Here's how the part is built. I have some questions about the finished solid (model axes, mm). A direction names the side the tool comes from. Round coordinates to 2 decimals unless told otherwise and drop trailing zeros. Order: outer loops, then holes, each group sorted by start corner. A loop starts at its lowest first (then second) coordinate and runs counter-clockwise, first axis right, second up. Notation, with made-up numbers: M -36.75,4.5 L 6.25,4.5 A19 cw 6.25,28.5 Z; hole C -28,48.5 d9. An arc over 180 degrees is marked long. Write each question's results on one line, items separated by ' | '. Start each with the question number.
```python
from build123d import *

# Parameters (mm, degrees)
EXTRUDE_1_DEPTH          = 2
SKETCH_1_3_W             = 2.1
SKETCH_1_3_H             = 8.1
CUT_EXTRUDE_1_DEPTH      = 31.615900009
SKETCH_2_R               = 1.55
SKETCH_2_R_2             = 6
CUT_EXTRUDE_2_DEPTH      = 10
FILLET_1_R               = 10
SKETCH_4_R               = 0.4
CUT_EXTRUDE_3_DEPTH      = 10
PATTERN_CIRCULAR_1_COUNT = 5
PATTERN_CIRCULAR_1_ANGLE = 240
FILLET_2_R               = 0.3


with BuildPart() as part:
    # 草图1 → 凸台-拉伸1 (new body)
    with BuildSketch(Plane(origin=(0, 0, 0), x_dir=(1, 0, 0), z_dir=(0, 1, 0))):
        Polygon((20, -11.547005384), (20, 11.547005384), (0, 23.094010768), (-20, 11.547005384), (-20, -11.547005384), (0, -23.094010768), align=None)
    extrude(amount=EXTRUDE_1_DEPTH)

    # 草图1<3> → 切除-拉伸1 (cut, through all)
    with BuildSketch(Plane(origin=(0, 0, 0), x_dir=(1, 0, 0), z_dir=(0, 1, 0))):
        Polygon((8.091952768, -5.884326674), (15.106758538, -9.934326674), (16.156758538, -8.115673326), (9.141952768, -4.065673326), align=None)
        with Locations((0, -14)):
            Rectangle(SKETCH_1_3_W, SKETCH_1_3_H)
        Polygon((-8.091952768, -5.884326674), (-15.106758538, -9.934326674), (-16.156758538, -8.115673326), (-9.141952768, -4.065673326), align=None)
        Polygon((-9.141952768, 4.065673326), (-16.156758538, 8.115673326), (-15.106758538, 9.934326674), (-8.091952768, 5.884326674), align=None)
        Polygon((8.091952768, 5.884326674), (15.106758538, 9.934326674), (16.156758538, 8.115673326), (9.141952768, 4.065673326), align=None)
    extrude(amount=CUT_EXTRUDE_1_DEPTH, mode=Mode.SUBTRACT)

    # 草图2 → 切除-拉伸2 (cut)
    with BuildSketch(Plane(origin=(0, 2, 0), x_dir=(1, 0, 0), z_dir=(0, 1, 0))):
        with Locations(Location((15, 0, 0), (0, 0, 270))):
            Circle(SKETCH_2_R)
        with Locations(Location((0, 0, 0), (0, 0, 270))):
            Circle(SKETCH_2_R_2)
        with Locations(Location((7.5, -12.990381057, 0), (0, 0, 270))):
            Circle(SKETCH_2_R)
        with Locations(Location((-7.5, -12.990381057, 0), (0, 0, 270))):
            Circle(SKETCH_2_R)
        with Locations(Location((-15, 0, 0), (0, 0, 270))):
            Circle(SKETCH_2_R)
        with Locations(Location((-7.5, 12.990381057, 0), (0, 0, 270))):
            Circle(SKETCH_2_R)
        with Locations(Location((7.5, 12.990381057, 0), (0, 0, 270))):
            Circle(SKETCH_2_R)
    extrude(amount=-CUT_EXTRUDE_2_DEPTH, mode=Mode.SUBTRACT)

    # 圆角1
    fillet_1_edges = [part.edges().sort_by_distance(p)[0] for p in [
        (20, 1, -11.547005384),
        (20, 1, 11.547005384),
        (0, 1, 23.094010768),
        (-20, 1, 11.547005384),
        (-20, 1, -11.547005384),
        (0, 1, -23.094010768),
    ]]
    fillet(fillet_1_edges, radius=FILLET_1_R)

    # 草图4 → 切除-拉伸3 (cut)
    with BuildSketch(Plane(origin=(0, 2, 0), x_dir=(1, 0, 0), z_dir=(0, 1, 0))):
        with Locations((15.00323092, 9.547956343)):
            Circle(SKETCH_4_R)
        with Locations((15.770388208, 8.219200944)):
            Circle(SKETCH_4_R)
        with Locations((8.478323098, 5.780799056)):
            Circle(SKETCH_4_R)
        with Locations((9.245480386, 4.452043657)):
            Circle(SKETCH_4_R)
    cut_extrude_3 = extrude(amount=-CUT_EXTRUDE_3_DEPTH, mode=Mode.SUBTRACT)

    # 阵列(圆周)1: 切除-拉伸3 ×5 about axis
    pattern_circular_1_axis = Axis((0, 0, 0), (0, -1, 0))
    for i in range(1, PATTERN_CIRCULAR_1_COUNT):
        add(cut_extrude_3.rotate(pattern_circular_1_axis, i * PATTERN_CIRCULAR_1_ANGLE / (PATTERN_CIRCULAR_1_COUNT - 1)), mode=Mode.SUBTRACT)

    # 圆角2
    fillet_2_edges = [part.edges().sort_by_distance(p)[0] for p in [
        (8.37479548, 1, -5.394428725),
        (8.859110055, 1, -4.555571275),
        (14.61686059, 1, -9.651483961),
        (15.873915826, 1, -8.605571275),
        (15.389601251, 1, -9.444428725),
        (15.66686059, 1, -7.832830614),
        (9.631850716, 1, -4.348516039),
        (8.581850716, 1, -6.167169386),
        (-8.859110055, 1, -4.555571275),
        (-8.37479548, 1, -5.394428725),
        (-15.66686059, 1, -7.832830614),
        (-15.389601251, 1, -9.444428725),
        (-8.859110055, 1, 4.555571275),
        (-8.37479548, 1, 5.394428725),
        (-14.61686059, 1, 9.651483961),
        (-15.873915826, 1, 8.605571275),
        (-0.484314575, 1, 9.95),
        (0.484314575, 1, 9.95),
        (1.05, 1, 17.484314575),
        (-0.484314575, 1, 18.05),
        (15.873915826, 1, 8.605571275),
        (15.389601251, 1, 9.444428725),
        (8.581850716, 1, 6.167169386),
        (8.859110055, 1, 4.555571275),
        (-14.61686059, 1, -9.651483961),
        (-15.873915826, 1, -8.605571275),
        (14.61686059, 1, 9.651483961),
        (15.66686059, 1, 7.832830614),
        (8.37479548, 1, 5.394428725),
        (1.05, 1, 10.515685425),
        (-1.05, 1, 10.515685425),
        (0.484314575, 1, 18.05),
        (-8.581850716, 1, -6.167169386),
        (-9.631850716, 1, -4.348516039),
        (-15.66686059, 1, 7.832830614),
        (-1.05, 1, 17.484314575),
        (-8.581850716, 1, 6.167169386),
        (-9.631850716, 1, 4.348516039),
        (-15.389601251, 1, 9.444428725),
        (9.631850716, 1, 4.348516039),
    ]]
    fillet(fillet_2_edges, radius=FILLET_2_R)


solid = part.part
```
(1) If we mould it in two halves opening along Z, with no side actions, what happens to faces 1 (the flat face through (12.69, 0.986, -6.114)), 2 (the flat face through (-20, 1, 0)), 3 (the flat face through (10.07, 0.99, -17.28))? For each: pulls with the +Z half, pulls with the -Z half, needs draft (parallel to the pull), parting line crosses it, or undercut.
(2) On a 3-axis mill with a long thin cutter (end or side, diameter ignored), from which of +Z, -Z, +X, -X, +Y, -Y can I reach the whole of each face in a straight line? I mean faces 4 (the flat face through (11.558, 0.986, -7.886)), 5 (the flat face through (-10.07, 0.99, 17.28)). Say none if no direction works.
(3) Please list where these lines run through material, in increasing order: line 1 (X direction, y = 1.3, z = 0); line 2 (X direction, y = 0.6, z = -4); line 3 (X direction, y = 1.4, z = -8.5).
(4) I want a section at A-A on z = 0. Write out the boundary of the cut face in (x, y).
(5) I want a section at D-D on x = -4.5. Write out the boundary of the cut face in (y, z), and give its area (3 significant figures).
(6) I want a section at B-B on z = -13.5. Write out the boundary of the cut face in (x, y).
(7) I'm going to push flat-ended pins straight in: pin 1 Ø1.9 at (x, z) = (-15, 0) entering from +Y; pin 2 Ø0.6 at (y, z) = (1.5, 14.5) entering from +X. Where does each tip first touch, or does it pass through?
(8) I want a section at C-C on x = 7.5. Write out the boundary of the cut face in (y, z).
Solutions:
1) face 1: undercut | face 2: needs draft | face 3: pulls with the -Z half
2) face 4: +Y, -Y | face 5: +Z, -X, +Y, -Y
3) line 1: -20 to -16.55, -13.45 to -6, 6 to 13.45, 16.55 to 20 | line 2: -20 to -4.47, 4.47 to 20 | line 3: -19.62 to -16.06, -12.62 to 12.62, 16.06 to 19.62
4) outline: M -20,0 L -16.55,0 L -16.55,2 L -20,2 Z; M -13.45,0 L -6,0 L -6,2 L -13.45,2 Z; M 6,0 L 13.45,0 L 13.45,2 L 6,2 Z; M 16.55,0 L 20,0 L 20,2 L 16.55,2 Z
5) outline: M 0,-20.48 L 2,-20.48 L 2,-3.97 L 0,-3.97 Z; M 0,3.97 L 2,3.97 L 2,20.48 L 0,20.48 Z | area: 66.0 mm^2
6) outline: M -16.35,0 L -8.96,0 L -8.96,2 L -16.35,2 Z; M -6.04,0 L 6.04,0 L 6.04,2 L -6.04,2 Z; M 8.96,0 L 16.35,0 L 16.35,2 L 8.96,2 Z
7) pin 1: through | pin 2: x = 15.38
8) outline: M 0,-18.76 L 2,-18.76 L 2,-14.54 L 0,-14.54 Z; M 0,-11.44 L 2,-11.44 L 2,11.44 L 0,11.44 Z; M 0,14.54 L 2,14.54 L 2,18.76 L 0,18.76 Z
